from build123d import *

# Parameters (mm, degrees)
F1_DEPTH  = 25.4
F3_DEPTH  = 50.801
F4_W      = 25.4
F4_H      = 12.7
F5_DEPTH  = 25.4
F6_W      = 25.4
F6_H      = 50.8
F7_DEPTH  = 25.4
F8_W      = 12.7
F8_H      = 25.4
F9_DEPTH  = 12.7
F10_DEPTH = 50.801
F12_DEPTH = 76.201


with BuildPart() as f1:
    # F0 (on Top) → F1 (new body, symmetric)
    with BuildSketch(Plane.XY):
        with BuildLine():
            Line((0, 50.8), (0, 0))
            Line((0, 0), (76.2, 0))
            Line((76.2, 0), (76.2, 39.1281142461))
            ThreePointArc((76.2, 39.1281142461), (72.7813838119, 47.3813838119), (64.5281142461, 50.8))
            Line((64.5281142461, 50.8), (0, 50.8))
        make_face()
    extrude(amount=F1_DEPTH, both=True)

    # F2 (on face) → F3 (cut, through all)
    with BuildSketch(Plane.XZ):
        Polygon((12.7, 25.4), (0, 25.4), (0, 12.7), align=None)
    extrude(amount=-F3_DEPTH, mode=Mode.SUBTRACT)

    # F4 (on face) → F5 (cut)
    with BuildSketch(Plane.XY.offset(25.4)):
        with Locations((38.1, 44.45)):
            Rectangle(F4_W, F4_H)
        with Locations((38.1, 6.35)):
            Rectangle(F4_W, F4_H)
    extrude(amount=-F5_DEPTH, mode=Mode.SUBTRACT)

    # F6 (on face) → F7 (cut, through all)
    with BuildSketch(Plane.XY.offset(25.4)):
        with Locations((63.5, 25.4)):
            Rectangle(F6_W, F6_H)
    extrude(amount=-F7_DEPTH, mode=Mode.SUBTRACT)

    # F8 (on face) → F9 (cut)
    with BuildSketch(Plane.XY.offset(25.4)):
        with Locations((44.45, 25.4)):
            Rectangle(F8_W, F8_H)
    extrude(amount=-F9_DEPTH, mode=Mode.SUBTRACT)

    # F4 (on face) → F10 (cut, through all)
    with BuildSketch(Plane.XY.offset(25.4)):
        with BuildLine():
            Line((76.2, 0), (76.2, 12.7))
            ThreePointArc((76.2, 12.7), (72.4802561211, 3.7197438789), (63.5, 0))
            Line((63.5, 0), (76.2, 0))
        make_face()
    extrude(amount=-F10_DEPTH, mode=Mode.SUBTRACT)

    # F11 (on face) → F12 (cut, through all)
    with BuildSketch(Plane.YZ.offset(76.2)):
        with BuildLine():
            Line((19.564057123, 0), (32.264057123, 0))
            ThreePointArc((32.264057123, 0), (25.914057123, 6.35), (19.564057123, 0))
        make_face()
        with BuildLine():
            ThreePointArc((19.564057123, 0), (25.914057123, -6.35), (32.264057123, 0))
            Line((32.264057123, 0), (19.564057123, 0))
        make_face()
    extrude(amount=-F12_DEPTH, mode=Mode.SUBTRACT)


solid = f1.part
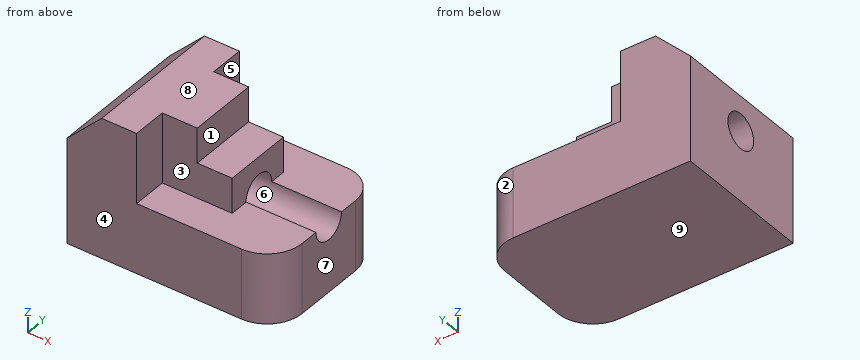
Can you work these out from the model? Positions are in its coordinate system, mm. Face numbers are marked on the shaded views. A direction names the side the tool comes from. Round coordinates to 2 decimals unless told otherwise and drop trailing zeros. Write each loop counter-clockwise with the first axis right and the second up, starting at its lowest first coordinate (ties: lowest second). Pieces come first, ordered by that corner, then holes. Notation, with made-up numbers: (67, 74) -> (112, 74) arc R14 ccw to (112, 95) -> close; hole circle Ø8 at (33, 78). An arc over 180 degrees is marked (long way). One line per question, with ' | ' between items. Start each with the question number.
1) Suppose I cut it at C-C on z = 20. Write out the boundary of the cut face in (x, y), then the cut area to 3 significant figures.
2) Suppose I cut it at B-B on y = 22.5. Write out the boundary of the cut face in (x, z), then the cut area to 3 significant figures.
3) I'm going to push flat-ended pins straight in: P1, Ø6, axis at x = 48.5, y = 13, coming from the +Z side; P2, Ø12.5, axis at x = 39, z = 14, coming from the -Y side; P3, Ø6.5, axis at y = 45.5, z = 15.5, coming from the +X side. Where does each tip first touch, or does it pass through?
4) If we mould it in two halves opening along Z, with no side actions, what happens to the marked faces 6, 7, 8 and 9? For each: released by +Z, released by -Z, zero draft, split by the parting line, or undercut.
5) I need wall thicknesses on line 1 (X direction, y = 38, z = 2); line 2 (Y direction, x = 29.5, z = 12.5); line 3 (Z direction, x = 29, y = 29). Which ranges of each line are inside material? Lowest first, please. Write a range as [from, to].
6) Suppose I cut it at A-A on x = 33. Write out the boundary of the cut face in (y, z), then the cut area to 3 significant figures.
7) Suppose I cut it at D-D on z = -1.5. Write out the boundary of the cut face in (x, y), then the cut area to 3 significant figures.
8) On a 3-axis mill with a long thin cutter (end or side, diameter ignored), from which of +Z, -Z, +X, -X, +Y, -Y can I reach the whole of each face in a straight line? I mean the marked faces 1, 2, 3, 4 and 5. Say none if no direction works.
Return value:
1) outline: (7.3, 0) -> (25.4, 0) -> (25.4, 12.7) -> (38.1, 12.7) -> (38.1, 38.1) -> (25.4, 38.1) -> (25.4, 50.8) -> (7.3, 50.8) -> close | area: 1,240 mm2
2) outline: (0, -25.4) -> (76.2, -25.4) -> (76.2, -5.35) -> (0, -5.35) -> close; (0, 5.35) -> (50.8, 5.35) -> (50.8, 12.7) -> (38.1, 12.7) -> (38.1, 25.4) -> (12.7, 25.4) -> (0, 12.7) -> close | area: 2,300 mm2
3) P1: stops at z = 12.7 | P2: stops at y = 12.7 | P3: stops at x = 25.4
4) face 6: undercut | face 7: zero draft | face 8: released by +Z | face 9: released by -Z
5) line 1: x = [0, 50.8] | line 2: y = [12.7, 38.1] | line 3: z = [-25.4, -5.55], [5.55, 25.4]
6) outline: (0, -25.4) -> (50.8, -25.4) -> (50.8, 0) -> (38.1, 0) -> (38.1, 25.4) -> (12.7, 25.4) -> (12.7, 0) -> (0, 0) -> close; hole circle Ø12.7 at (25.91, 0) | area: 1,810 mm2
7) outline: (0, 0) -> (63.5, 0) arc R12.7 ccw to (76.2, 12.7) -> (76.2, 19.74) -> (0, 19.74) -> close; (0, 32.08) -> (76.2, 32.08) -> (76.2, 39.13) arc R11.67 ccw to (64.53, 50.8) -> (0, 50.8) -> close | area: 2,870 mm2
8) face 1: +Z, +X, +Y, -Y | face 2: +Z, -Z, +X, +Y | face 3: +Z, +X, -Y | face 4: +Z, -Z, +X, -X, -Y | face 5: +Z, +X, +Y
